```python
from build123d import *

# Parameters (mm, degrees)
SKETCH_1_W          = 54
SKETCH_1_H          = 34
EXTRUDE_1_DEPTH     = 1500
SKETCH_2_R          = 4.05
CUT_EXTRUDE_1_DEPTH = 41


with BuildPart() as part:
    # Эскиз1 → Вытянуть-Тонкостенный1 (new body)
    with BuildSketch(Plane(origin=(0, 0, 0), x_dir=(0, 0, -1), z_dir=(1, 0, 0))):
        with BuildLine():
            Line((30, 17), (30, -17))
            ThreePointArc((30, -17), (29.121320344, -19.121320344), (27, -20))
            Line((27, -20), (-27, -20))
            ThreePointArc((-27, -20), (-29.121320344, -19.121320344), (-30, -17))
            Line((-30, -17), (-30, 17))
            ThreePointArc((-30, 17), (-29.121320344, 19.121320344), (-27, 20))
            Line((-27, 20), (27, 20))
            ThreePointArc((27, 20), (29.121320344, 19.121320344), (30, 17))
        make_face()
        Rectangle(SKETCH_1_W, SKETCH_1_H, mode=Mode.SUBTRACT)
    extrude(amount=EXTRUDE_1_DEPTH)

    # Эскиз2 → Вырез-Вытянуть1 (cut, through all)
    with BuildSketch(Plane(origin=(0, 20, 0), x_dir=(1, 0, 0), z_dir=(0, 1, 0))):
        with Locations((1455, -12)):
            Circle(SKETCH_2_R)
        with Locations((1405, -12)):
            Circle(SKETCH_2_R)
        with Locations((1355, -12)):
            Circle(SKETCH_2_R)
        with Locations((1305, -12)):
            Circle(SKETCH_2_R)
        with Locations((1155, -12)):
            Circle(SKETCH_2_R)
        with Locations((1105, -12)):
            Circle(SKETCH_2_R)
        with Locations((1055, -12)):
            Circle(SKETCH_2_R)
        with Locations((1005, -12)):
            Circle(SKETCH_2_R)
    extrude(amount=-CUT_EXTRUDE_1_DEPTH, mode=Mode.SUBTRACT)


solid = part.part
```
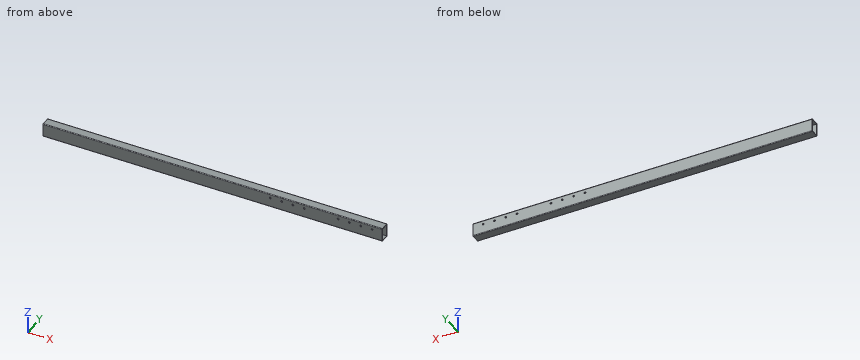
Design review of the part built by this model. Coordinates are the model's own, in mm. Round coordinates to 2 decimals unless told otherwise and drop trailing zeros. Order: outer loops, then holes, each group sorted by start corner. A loop starts at its lowest first (then second) coordinate and runs counter-clockwise, first axis right, second up. Notation, with made-up numbers: (-36.5, 41) - (-18.5, 41) arc R20 ccw to (-18.5, 76) - close; hole circle Ø11 at (-37, 39). An arc over 180 degrees is marked (long way). Return JSON: item names as keys, results as strings.
Q1. Wall thickness on L1, parallel to Z at x = 475, y = 0.5; L2, parallel to Y at x = 167.5, z = -7; L3, parallel to Z at x = 1055, y = -17.95: over which ranges is each line inside the solid? List them lowest first. Write a range as [from, to].
Computed values:
{"L1": "z = [-30, -27], [27, 30]", "L2": "y = [-20, -17], [17, 20]", "L3": "z = [-29.85, 7.95], [16.05, 29.85]"}
Q2. For pin 1 Ø6.5 at (x, z) = (1155, 12) entering from -Y, flat-tipped, find the tip position at first contact; note if it passes through.
Computed values:
{"pin 1": "passes through"}
Q3. Consider section C-C on y = 1.5. Write out the cut boundary in (x, z), plus the area to 3 significant figures.
Computed values:
{"outline": "(0, -30) - (1500, -30) - (1500, -27) - (0, -27) - close; (0, 27) - (1500, 27) - (1500, 30) - (0, 30) - close", "area": "9,000 mm2"}
Q4. Consider section B-B on z = -3. Write out the cut boundary in (x, y).
Computed values:
{"outline": "(0, -20) - (1500, -20) - (1500, -17) - (0, -17) - close; (0, 17) - (1500, 17) - (1500, 20) - (0, 20) - close"}
Q5. Consider section A-A on x = 931.5. Write out the cut boundary in (y, z).
Computed values:
{"outline": "(-20, -27) arc R3 ccw to (-17, -30) - (17, -30) arc R3 ccw to (20, -27) - (20, 27) arc R3 ccw to (17, 30) - (-17, 30) arc R3 ccw to (-20, 27) - close; hole (-17, -27) - (17, -27) - (17, 27) - (-17, 27) - close"}
